Source: CAD feature listing. Evaluate the final solid. Frame: model axes, mm. A direction names the side the tool comes from. Coordinates: 2 decimals unless noted, no trailing zeros. Order: outer loops, then holes, each group sorted by start corner. A loop starts at its lowest first (then second) coordinate and runs counter-clockwise, first axis right, second up. Notation, with made-up numbers: (37, -5) -> (68, -5) arc R20 cw to (68, 2) -> close; hole circle Ø1 at (-35.75, 88). An arc over 180 degrees is marked (long way). Put each result on its own line as item: value.
from build123d import *

# Parameters (mm, degrees)
BOSS_EXTRUDE2_DEPTH   = 144
BOSS_EXTRUDE2_2_DEPTH = 144
BOSS_EXTRUDE3_START   = 118
BOSS_EXTRUDE3_DEPTH   = 26
BOSS_EXTRUDE4_DEPTH   = 22
CHAMFER1_SIZE         = 16


# Read off the part's stored shape, not the designer's step: Ø2.0 (6) Diameter Hole1
with BuildPart() as part:
    # Sketch1 → Boss-Extrude2 (new body)
    with BuildSketch(Plane.XY):
        Polygon((26.980199866, -10), (8, -10), (8, -19), (16, -19), (16, -26), (32, -26), (32, -10), align=None)
    extrude(amount=BOSS_EXTRUDE2_DEPTH)



with BuildPart() as body_2:
    # Sketch1 → Boss-Extrude2 2 (new body)
    with BuildSketch(Plane.XY):
        Polygon((-32, -10), (-32, -26), (-16, -26), (-16, -19), (-8, -19), (-8, -10), (-26.980199866, -10), align=None)
    extrude(amount=BOSS_EXTRUDE2_2_DEPTH)


with BuildPart() as part_1:
    add(part.part)

    add(body_2.part)  # Boss-Extrude3 merges body 2
    # Sketch1<5> → Boss-Extrude3 (add)
    with BuildSketch(Plane.XY.offset(BOSS_EXTRUDE3_START)):
        Polygon((17.654046703, 10), (26.980199866, -10), (32, -10), (32, 10), align=None)
        with BuildLine():
            Line((32, 26), (-2.1e-08, 26))
            ThreePointArc((-2.1e-08, 26), (8.596793725, 23.494263139), (14.500924593, 16.761892188))
            Line((14.500924593, 16.761892188), (17.654046703, 10))
            Line((17.654046703, 10), (32, 10))
            Line((32, 10), (32, 26))
        make_face()
        with BuildLine():
            Line((-32, 26), (-32, 10))
            Line((-32, 10), (-17.654046703, 10))
            Line((-17.654046703, 10), (-14.500924593, 16.761892188))
            ThreePointArc((-14.500924593, 16.761892188), (-8.596793742, 23.494263127), (-2.1e-08, 26))
            Line((-2.1e-08, 26), (-32, 26))
        make_face()
        with BuildLine():
            Line((-14.500924593, 16.761892188), (-17.654046703, 10))
            Line((-17.654046703, 10), (-8, 10))
            ThreePointArc((-8, 10), (0, 18), (8, 10))
            Line((8, 10), (17.654046703, 10))
            Line((17.654046703, 10), (14.500924593, 16.761892188))
            ThreePointArc((14.500924593, 16.761892188), (8.596793725, 23.494263139), (-2.1e-08, 26))
            ThreePointArc((-2.1e-08, 26), (-8.596793742, 23.494263127), (-14.500924593, 16.761892188))
        make_face()
        with BuildLine():
            Line((-17.654046703, 10), (-26.980199866, -10))
            Line((-26.980199866, -10), (-8, -10))
            Line((-8, -10), (8, -10))
            Line((8, -10), (26.980199866, -10))
            Line((26.980199866, -10), (17.654046703, 10))
            Line((17.654046703, 10), (8, 10))
            ThreePointArc((8, 10), (0, 2), (-8, 10))
            Line((-8, 10), (-17.654046703, 10))
        make_face()
        with BuildLine():
            ThreePointArc((8, 10), (0, 18), (-8, 10))
            Line((-8, 10), (8, 10))
        make_face()
        with BuildLine():
            Line((8, 10), (-8, 10))
            ThreePointArc((-8, 10), (0, 2), (8, 10))
        make_face()
        Polygon((-32, 10), (-32, -10), (-26.980199866, -10), (-17.654046703, 10), align=None)
        Polygon((-32, -10), (-32, -26), (-16, -26), (-16, -19), (-8, -19), (-8, -10), (-26.980199866, -10), align=None)
        Polygon((26.980199866, -10), (8, -10), (8, -19), (16, -19), (16, -26), (32, -26), (32, -10), align=None)
    extrude(amount=BOSS_EXTRUDE3_DEPTH)

    # Sketch1<6> → Boss-Extrude4 (add)
    with BuildSketch(Plane.XY):
        with BuildLine():
            Line((-17.654046703, 10), (-26.980199866, -10))
            Line((-26.980199866, -10), (-8, -10))
            Line((-8, -10), (8, -10))
            Line((8, -10), (26.980199866, -10))
            Line((26.980199866, -10), (17.654046703, 10))
            Line((17.654046703, 10), (8, 10))
            ThreePointArc((8, 10), (0, 2), (-8, 10))
            Line((-8, 10), (-17.654046703, 10))
        make_face()
        with BuildLine():
            Line((-14.500924593, 16.761892188), (-17.654046703, 10))
            Line((-17.654046703, 10), (-8, 10))
            ThreePointArc((-8, 10), (0, 18), (8, 10))
            Line((8, 10), (17.654046703, 10))
            Line((17.654046703, 10), (14.500924593, 16.761892188))
            ThreePointArc((14.500924593, 16.761892188), (8.596793725, 23.494263139), (-2.1e-08, 26))
            ThreePointArc((-2.1e-08, 26), (-8.596793742, 23.494263127), (-14.500924593, 16.761892188))
        make_face()
    extrude(amount=BOSS_EXTRUDE4_DEPTH)

    # Chamfer1
    chamfer1_edges = [part_1.edges().sort_by_distance(p)[0] for p in [
        (0, 26, 144),
    ]]
    chamfer(chamfer1_edges, length=CHAMFER1_SIZE)

    # Ø2.0 (6) Diameter Hole1 outline → Ø2.0 (6) Diameter Hole1 (revolve, cut)
    with BuildSketch(Plane(origin=(-22, 0, 38), x_dir=(1, 0, 0), z_dir=(0, 0, 1))):
        Polygon((3, -16), (0, -14.267949192), (0, -26), (3, -26), align=None)
    revolve(axis=Axis((-22, 0, 38), (0, 1, 0)), mode=Mode.SUBTRACT)

    # 2.0 _6_ Diameter Hole1 2 outline → 2.0 _6_ Diameter Hole1 2 (revolve, cut)
    with BuildSketch(Plane(origin=(22, 0, 108), x_dir=(1, 0, 0), z_dir=(0, 0, 1))):
        Polygon((3, -16), (0, -14.267949192), (0, -26), (3, -26), align=None)
    revolve(axis=Axis((22, 0, 108), (0, 1, 0)), mode=Mode.SUBTRACT)

    # 2.0 _6_ Diameter Hole1 3 outline → 2.0 _6_ Diameter Hole1 3 (revolve, cut)
    with BuildSketch(Plane(origin=(-22, 0, 108), x_dir=(1, 0, 0), z_dir=(0, 0, 1))):
        Polygon((3, -16), (0, -14.267949192), (0, -26), (3, -26), align=None)
    revolve(axis=Axis((-22, 0, 108), (0, 1, 0)), mode=Mode.SUBTRACT)

    # 2.0 _6_ Diameter Hole1 4 outline → 2.0 _6_ Diameter Hole1 4 (revolve, cut)
    with BuildSketch(Plane(origin=(22, 0, 38), x_dir=(1, 0, 0), z_dir=(0, 0, 1))):
        Polygon((3, -16), (0, -14.267949192), (0, -26), (3, -26), align=None)
    revolve(axis=Axis((22, 0, 38), (0, 1, 0)), mode=Mode.SUBTRACT)


solid = part_1.part
1. Cut plane B-B on z = 123.5. Output: boundary loops of the cut face in (x, y).
Numbers:
outline: (-32, -26) -> (-16, -26) -> (-16, -19) -> (-8, -19) -> (-8, -10) -> (8, -10) -> (8, -19) -> (16, -19) -> (16, -26) -> (32, -26) -> (32, 26) -> (-32, 26) -> close
2. Set-up query: faces 1 (the flat face through (0, -10, 11)), 2 (the cylindrical face through (1.73, 2.19, 10.85)), 3 (the flat face through (0, 0, 22)), 4 (the flat face through (0, 18, 136)). Return all of +Z, -Z, +X, -X, +Y, -Y with unobstructed straight access to the full face (end or side cutting, diameter ignored); none if empty.
Numbers:
face 1: +Z, -Z, -Y
face 2: -Z
face 3: +X, -X, +Y
face 4: +Z, +X, -X, +Y
3. Ray query, line 1 along X through (y, z) = (-20.5, 38); line 2 along Z through (x, y) = (-22, -20); line 3 along X through (y, z) = (-20, 12.5). Return the intervals inside material, ascending.
Numbers:
line 1: x = -32 to -25, -19 to -16, 16 to 19, 25 to 32
line 2: z = 0 to 35, 41 to 105, 111 to 144
line 3: x = -32 to -16, 16 to 32
4. First-contact query: pin 1 (12 mm diameter, centred on x = 15, z = 58, fed in from +Y); pin 2 (1 mm diameter, centred on x = -12.5, z = 56, fed in from -Y); pin 3 (8 mm diameter, centred on x = 2.5, z = 132, fed in from -Y); pin 4 (8 mm diameter, centred on x = -1, z = 107, fed in from +Y). Flat tips, straight axial feed; report the tip coordinate or a pass-through.
Numbers:
pin 1: stops at y = -10
pin 2: stops at y = -19
pin 3: stops at y = -10
pin 4: passes through
5. Cut plane C-C on x = -9.5. Output: boundary loops of the cut face in (y, z), plus the area to 3 significant figures.
Numbers:
outline: (-19, 0) -> (22.87, 0) -> (22.87, 22) -> (-10, 22) -> (-10, 118) -> (26, 118) -> (26, 128) -> (10, 144) -> (-19, 144) -> close
area: 2,830 mm2
6. Cut plane A-A on z = 30. Output: boundary loops of the cut face in (x, y), plus the area to 3 significant figures.
Numbers:
outline: (-32, -26) -> (-16, -26) -> (-16, -19) -> (-8, -19) -> (-8, -10) -> (-32, -10) -> close; (8, -19) -> (16, -19) -> (16, -26) -> (32, -26) -> (32, -10) -> (8, -10) -> close
area: 656 mm2
7. Cut plane D-D on x = 13. Output: boundary loops of the cut face in (y, z).
Numbers:
outline: (-19, 0) -> (19.33, 0) -> (19.33, 22) -> (-10, 22) -> (-10, 118) -> (26, 118) -> (26, 128) -> (10, 144) -> (-19, 144) -> close
8. Pull-direction query (X, two-part tool) for faces 5 (the flat face through (32, -12, 87)), 6 (the flat face through (20, -10, 71)), 7 (the conical face through (22.22, -14.54, 38.42)); classes: pulls with the +X half, pulls with the -X half, needs draft (parallel to the pull), parting line crosses it, or undercut.
Numbers:
face 5: pulls with the +X half
face 6: needs draft
face 7: undercut
